from build123d import *

# Parameters (mm, degrees)
BOSS_EXTRUDE1_DEPTH                             = 281.94
BOSS_EXTRUDE1_DEPTH_BACK                        = 276.86
CBORE_FOR_M4_SHCS1_D                            = 4.5
CBORE_FOR_M4_SHCS1_CBORE_D                      = 8
CBORE_FOR_M4_SHCS1_CBORE_DEPTH                  = 4
CSK_FOR_M4_FLAT_HEAD_MACHINE_SCREW1_D           = 4.5
CSK_FOR_M4_FLAT_HEAD_MACHINE_SCREW1_CSINK_D     = 9.4
CSK_FOR_M4_FLAT_HEAD_MACHINE_SCREW1_CSINK_ANGLE = 90
LPATTERN1_COUNT                                 = 9
LPATTERN1_PITCH                                 = 60
LPATTERN1_COL_COUNT                             = 2
LPATTERN1_COL_PITCH                             = 60
F_6_32_TAPPED_HOLE1_D                           = 2.7051


with BuildPart() as part:
    # Sketch1 → Boss-Extrude1 (new, two sides: drawn at the far end of the back side and taken through both)
    with BuildSketch(Plane.XY.offset(-BOSS_EXTRUDE1_DEPTH_BACK)):
        Polygon((-39.1, 20), (-39.1, 11.75), (-40.375, 11.75), (-40.375, 18), (-44.875, 18), (-44.875, 6.25), (-41.875, 6.25), (-41.875, 5.5), (-43.125, 4.778312164), (-43.125, -4.778312164), (-41.875, -5.5), (-41.875, -6.25), (-44.875, -6.25), (-44.875, -18), (-40.375, -18), (-40.375, -11.75), (-39.1, -11.75), (-39.1, -20), (-47.625, -20), (-47.625, 20), align=None)
    extrude(amount=BOSS_EXTRUDE1_DEPTH + BOSS_EXTRUDE1_DEPTH_BACK)

    # CBORE for M4 SHCS1 (through all)
    with Locations(Plane(origin=(-43.125, 0, 0), x_dir=(0, 0, -1), z_dir=(1, 0, 0))):
        with Locations((-219.589999986, 0)):
            cbore_for_m4_shcs1 = CounterBoreHole(CBORE_FOR_M4_SHCS1_D / 2, CBORE_FOR_M4_SHCS1_CBORE_D / 2, CBORE_FOR_M4_SHCS1_CBORE_DEPTH)

    # CSK for M4 Flat Head Machine Screw1 (through all)
    with Locations(Plane(origin=(-47.625, 10.717833064, -20.25819937), x_dir=(0, 0, -1), z_dir=(-1, 0, 0))):
        with Locations((-260.84819952, 10.717833064), (-280.848199398, 10.717833064)):
            CounterSinkHole(CSK_FOR_M4_FLAT_HEAD_MACHINE_SCREW1_D / 2, CSK_FOR_M4_FLAT_HEAD_MACHINE_SCREW1_CSINK_D / 2, counter_sink_angle=CSK_FOR_M4_FLAT_HEAD_MACHINE_SCREW1_CSINK_ANGLE)

    # LPattern1: CBORE for M4 SHCS1 ×9
    with Locations(*[(0, 0, -i * LPATTERN1_PITCH) for i in range(1, LPATTERN1_COUNT)]):
        add(cbore_for_m4_shcs1, mode=Mode.SUBTRACT)

    # LPattern1 col: CBORE for M4 SHCS1 ×2
    with Locations(*[(0, 0, i * LPATTERN1_COL_PITCH) for i in range(1, LPATTERN1_COL_COUNT)]):
        add(cbore_for_m4_shcs1, mode=Mode.SUBTRACT)

    # #6-32 Tapped Hole1 (through all)
    with Locations(Plane(origin=(-44.875, 0, 0), x_dir=(0, 0, -1), z_dir=(1, 0, 0))):
        with Locations((273.685, -9.250000096), (273.685, 9.250000096)):
            Hole(F_6_32_TAPPED_HOLE1_D / 2)


solid = part.part
Geometry check sheet. Reference: the model listing, model coordinates, mm. A direction names the side the tool comes from. Give positions to 0.01 mm unless a question says otherwise; leave off trailing zeros. Write each loop counter-clockwise with the first axis right and the second up, starting at its lowest first coordinate (ties: lowest second). Pieces come first, ordered by that corner, then holes.
1) Release check for a two-part mould opening along Y. For faces 4 (the face through (-45.294, -0.712, 262.85)), 5 (the face through (-43, 20, -1)), 6 (the face through (-44.875, 12, -1)), 7 (the face through (-47.625, 0, -1)) record: released by +Y, released by -Y, zero draft, split by the parting line, or undercut.
Values follow:
face 4: undercut
face 5: released by +Y
face 6: undercut
face 7: zero draft
2) Go/stop test with flat-tipped pins: pin 1 Ø1.5 at (y, z) = (3, -63) entering from +X (3 decimals); pin 2 Ø4 at (y, z) = (1.5, -200) entering from +X (3 decimals); pin 3 Ø3.5 at (y, z) = (0, 279.59) entering from +X; pin 4 Ø1 at (y, z) = (-9.5, 210.5) entering from +X (3 decimals). Record where each tip stops, or that it passes through.
Values follow:
pin 1: stops at x = -43.125
pin 2: stops at x = -47.125
pin 3: passes through
pin 4: stops at x = -44.875
3) Cross-section at A-A (z = 8). Record the boundary of the cut face in (x, y) (3 decimals), plus the area to 3 significant figures.
Values follow:
outline: (-47.625, -20) - (-39.1, -20) - (-39.1, -11.75) - (-40.375, -11.75) - (-40.375, -18) - (-44.875, -18) - (-44.875, -6.25) - (-41.875, -6.25) - (-41.875, -5.5) - (-43.125, -4.778) - (-43.125, 4.778) - (-41.875, 5.5) - (-41.875, 6.25) - (-44.875, 6.25) - (-44.875, 18) - (-40.375, 18) - (-40.375, 11.75) - (-39.1, 11.75) - (-39.1, 20) - (-47.625, 20) - close
area: 174 mm2
4) Set-up check for faces 1 (the face through (-43.125, 0, -1)), 2 (the face through (-44.875, -12, -1)), 3 (the face through (-45, 0, -276.86)): record each of +Z, -Z, +X, -X, +Y, -Y from which the full face is reachable in a straight line by a thin tool's end or side.
Values follow:
face 1: +Z, -Z, +X
face 2: +Z, -Z
face 3: -Z, +X, -X, +Y, -Y
5) Thickness scan on line 1 (Y direction, x = -44, z = 23.5); line 2 (Y direction, x = -41.75, z = 54.5); line 3 (Y direction, x = -45.8, z = -260.41). Record the ranges inside material, lowest first.
Values follow:
line 1: y = -20 to -18, -6.25 to 6.25, 18 to 20
line 2: y = -20 to -18, 18 to 20
line 3: y = -20 to -4, 4 to 20
